from build123d import *

# Parameters (mm, degrees)
SKETCH1_R           = 12.446
BOSS_EXTRUDE1_DEPTH = 12.7
CHAMFER1_SIZE       = 1.016
CHAMFER2_SIZE       = 1.016
SKETCH2_R           = 3.175
CUT_EXTRUDE1_DEPTH  = 25.4
CIRPATTERN4_COUNT   = 12


with BuildPart() as part:
    # Sketch1 → Boss-Extrude1 (new body, symmetric)
    with BuildSketch(Plane(origin=(0, 0, 0), x_dir=(0, 0, -1), z_dir=(1, 0, 0))):
        Circle(SKETCH1_R)
    extrude(amount=BOSS_EXTRUDE1_DEPTH, both=True)

    # Chamfer1
    chamfer1_edges = [part.edges().sort_by_distance(p)[0] for p in [
        (12.7, 0, 12.446),
    ]]
    chamfer(chamfer1_edges, length=CHAMFER1_SIZE)

    # Chamfer2
    chamfer2_edges = [part.edges().sort_by_distance(p)[0] for p in [
        (-12.7, 0, 12.446),
    ]]
    chamfer(chamfer2_edges, length=CHAMFER2_SIZE)

    # Sketch2 → Cut-Extrude1 (cut)
    with BuildSketch(Plane(origin=(12.7, 0, 0), x_dir=(0, 0, -1), z_dir=(1, 0, 0))):
        Circle(SKETCH2_R)
    extrude(amount=-CUT_EXTRUDE1_DEPTH, mode=Mode.SUBTRACT)

    # Sketch4 → #38 (0.1015) Diameter Hole1 (revolve, cut)
    with BuildSketch(Plane(origin=(0, 10.202452378, -7.128315472), x_dir=(0, 0.572739472, 0.819737456), z_dir=(1, 0, 0))):
        Polygon((0, 0), (0, 3.314539381), (1.28905, 2.54), (1.28905, 0), align=None)
    f_38_0_1015_diameter_hole1 = revolve(axis=Axis((0, 15.407785224, -10.765211121), (0, -0.819737456, 0.572739472)), mode=Mode.SUBTRACT)

    # CirPattern4: #38 (0.1015) Diameter Hole1 ×12 about axis
    cirpattern4_axis = Axis((12.7, 0, 0), (-1, 0, 0))
    for i in range(1, CIRPATTERN4_COUNT):
        add(f_38_0_1015_diameter_hole1.rotate(cirpattern4_axis, i * 360 / CIRPATTERN4_COUNT), mode=Mode.SUBTRACT)


solid = part.part
Can you work these out from the model? Positions are in its coordinate system, mm. A direction names the side the tool comes from. Coordinates: 2 decimals unless noted, no trailing zeros. Order: outer loops, then holes, each group sorted by start corner. A loop starts at its lowest first (then second) coordinate and runs counter-clockwise, first axis right, second up. Notation, with made-up numbers: (22.25, 86) - (65.25, 86) arc R28 cw to (65.25, 105) - close; hole circle Ø7 at (22, 26.5). An arc over 180 degrees is marked (long way). Answer as a JSON object with one key per item and string values. Group by question number.
Q1. We'd pull the mould along X, two halves only. Please class faces 1 (the face through (0.78, 10.57, 3.81)), 2 (the face through (-12.7, -2.4, -2.4)), 3 (the face through (12.7, -2.4, -2.4)): +X half, -X half, draft (parallel to the pull), parting line (faces both ways), or undercut.
Q2. Will these pins go through, and if not, where does the flat tip stop? P1, Ø10, axis at x = 3, y = 6.5, coming from the +Z side; P2, Ø2, axis at x = 0, z = -5, coming from the +Y side; P3, Ø3, axis at x = -6.5, y = -4.5, coming from the +Z side.
Q3. Imagine slicing it at A-A (x = -2). Please give me the cut outline in (y, z) (3 decimals), and give its area (3 significant figures).
Q4. I need wall thicknesses on line 1 (Y direction, x = 0.5, z = 0) (3 decimals); line 2 (Y direction, x = -5.75, z = 0) (3 decimals); line 3 (X direction, y = -5.75, z = -8.75). Which ranges of each line are inside material? Lowest first, please. Write a range as from..to.
Q5. On a 3-axis mill with a long thin cutter (end or side, diameter ignored), from which of +Z, -Z, +X, -X, +Y, -Y can I reach the whole of each face in a straight line? I mean faces 4 (the face through (0.16, -12.15, 2.7)), 5 (the face through (0, -5, -8)). Say none if no direction works.
Determined:
{
 "1": {"face 1": "undercut", "face 2": "-X half", "face 3": "+X half"},
 "2": {"P1": "stops at z = 12.36", "P2": "stops at y = 11.79", "P3": "stops at z = 12.08"},
 "3": {"outline": "circle Ø24.892 at (0, 0); hole circle Ø6.35 at (0, 0)", "area": "455 mm2"},
 "4": {"line 1": "y = -9.755..-3.175, 3.175..9.755", "line 2": "y = -12.446..-3.175, 3.175..12.446", "line 3": "x = -12.7..-1.25, 1.25..12.7"},
 "5": {"face 4": "+X, -X", "face 5": "none"}
}
